from build123d import *

# Parameters (mm, degrees)
SKETCH1_R           = 3
BOSS_EXTRUDE1_DEPTH = 3.7
SKETCH1_3_R         = 1.6
BOSS_EXTRUDE2_DEPTH = 1
SKETCH5_R           = 1.5
BOSS_EXTRUDE3_DEPTH = 1
SKETCH6_R           = 2
BOSS_EXTRUDE4_DEPTH = 1
SKETCH8_R           = 1.5
BOSS_EXTRUDE5_DEPTH = 2.5
SKETCH10_R          = 1.8
BOSS_EXTRUDE6_DEPTH = 1
SKETCH12_R          = 1.65
CUT_EXTRUDE1_DEPTH  = 2


with BuildPart() as part:
    # Sketch1 → Boss-Extrude1 (new body)
    with BuildSketch(Plane(origin=(0, 0, 0), x_dir=(1, 0, 0), z_dir=(0, 1, 0))):
        with Locations((-0.522013312, 0.511138034)):
            Circle(SKETCH1_R)
    extrude(amount=BOSS_EXTRUDE1_DEPTH)

    # Sketch1<3> → Boss-Extrude2 (add)
    with BuildSketch(Plane(origin=(0, 0, 0), x_dir=(1, 0, 0), z_dir=(0, 1, 0))):
        with Locations((-0.522013312, 0.511138034)):
            Circle(SKETCH1_3_R)
    extrude(amount=BOSS_EXTRUDE2_DEPTH)

    # Sketch5 → Boss-Extrude3 (add)
    with BuildSketch(Plane.XZ):
        with Locations((-0.522013312, -0.511138034)):
            Circle(SKETCH5_R)
    extrude(amount=BOSS_EXTRUDE3_DEPTH)

    # Sketch6 → Boss-Extrude4 (add)
    with BuildSketch(Plane.XZ.offset(1)):
        with Locations((-0.522013312, -0.511138034)):
            Circle(SKETCH6_R)
    extrude(amount=BOSS_EXTRUDE4_DEPTH)

    # Sketch8 → Boss-Extrude5 (add)
    with BuildSketch(Plane(origin=(0, -2, 0), x_dir=(-1, 0, 0), z_dir=(0, -1, 0))):
        with Locations((0.522013312, 0.511138034)):
            Circle(SKETCH8_R)
    extrude(amount=BOSS_EXTRUDE5_DEPTH)

    # Sketch10 → Boss-Extrude6 (add)
    with BuildSketch(Plane.XZ.offset(4.5)):
        with Locations((-0.522013312, -0.511138034)):
            Circle(SKETCH10_R)
    extrude(amount=-BOSS_EXTRUDE6_DEPTH)

    # Sketch12 → Cut-Extrude1 (cut)
    with BuildSketch(Plane(origin=(0, 3.7, 0), x_dir=(1, 0, 0), z_dir=(0, 1, 0))):
        with Locations((-0.522013312, 0.511138034)):
            Circle(SKETCH12_R)
    extrude(amount=-CUT_EXTRUDE1_DEPTH, mode=Mode.SUBTRACT)


solid = part.part
Model file for the job. Use its own axes, mm. A direction names the side the tool comes from. Give positions to 0.01 mm unless a question says otherwise; leave off trailing zeros. Loops run counter-clockwise (first coordinate to the right, second up) from the corner with the lowest first, then second, coordinate; pieces in that order, holes last. Notation, with made-up numbers: (24.25, 57.25) -> (50.25, 57.25) arc R17 cw to (50.25, 61.25) -> close; hole circle Ø5 at (0.5, 80.5). An arc over 180 degrees is marked (long way). Use a Markdown table: item, result. Add a question column.
(1) Slice it at D-D on y = -1.75. List the corners of the cut face in (x, z), and give its area (3 significant figures).
(2) Slice it at B-B on z = -1.9. List the corners of the cut face in (x, y).
(3) Drop flat-ended pins along their axis: pin 1 Ø1.6 at (x, z) = (-1, 0) entering from +Y; pin 2 Ø3 at (x, y) = (-3, 1.5) entering from +Z (3 decimals). Give the stop position or say it passes through.
(4) Wall check: line 1 along Y through (x, z) = (-1.9, 1.2); line 2 along X through (y, z) = (2.25, 0.3); line 3 along Y through (x, z) = (0.1, -1.5). Give the ranges that are in metal, low to high.
(5) Tool access for faces 1 (the flat face through (1, 3.7, 1)), 2 (the cylindrical face through (1.325, -1.493, -1.277)), 3 (the cylindrical face through (0.91, -0.49, -0.06)), 4 (the cylindrical face through (1.002, 2.714, 0.121)): list every direction of +Z, -Z, +X, -X, +Y, -Y with a clear straight run to the whole face (end or side of a thin tool).
(6) Slice it at C-C on y = 2.75. List the corners of the cut face in (x, z), and give its area (3 significant figures).
(7) Slice it at A-A on x = -0.25. List the corners of the cut face in (y, z), and give its area (3 significant figures).
(8) Mould opens along Z. For faces 5 (the flat face through (1, 0, 1)), 6 (the flat face through (-1, 1.7, -1)), 7 (the cylindrical face through (-0.197, -2.74, 0.953)) say: +Z half, -Z half, draft (parallel to the pull), parting line (faces both ways), or undercut.
Filled sheet:
| question | item | result |
|---|---|---|
| 1 | outline | circle Ø4 at (-0.52, -0.51) |
| 1 | area | 12.6 mm2 |
| 2 | outline | (-3.18, 0) -> (-1.09, 0) -> (-1.09, -1) -> (-1.96, -1) -> (-1.96, -2) -> (-1.09, -2) -> (-1.09, -3.5) -> (-1.67, -3.5) -> (-1.67, -4.5) -> (0.62, -4.5) -> (0.62, -3.5) -> (0.04, -3.5) -> (0.04, -2) -> (0.92, -2) -> (0.92, -1) -> (0.04, -1) -> (0.04, 0) -> (2.14, 0) -> (2.14, 3.7) -> (0.37, 3.7) -> (0.37, 1.7) -> (-1.41, 1.7) -> (-1.41, 3.7) -> (-3.18, 3.7) -> close |
| 3 | pin 1 | y = 1.7 |
| 3 | pin 2 | z = 2.325 |
| 4 | line 1 | 0 to 3.7 |
| 4 | line 2 | -3.41 to -1.96, 0.91 to 2.37 |
| 4 | line 3 | -4.5 to 1.7 |
| 5 | face 1 | +Z, -Z, +X, -X, +Y |
| 5 | face 2 | -Y |
| 5 | face 3 | none |
| 5 | face 4 | +Y |
| 6 | outline | circle Ø6 at (-0.52, -0.51); hole circle Ø3.3 at (-0.52, -0.51) |
| 6 | area | 19.7 mm2 |
| 7 | outline | (-4.5, -2.29) -> (-3.5, -2.29) -> (-3.5, -1.99) -> (-2, -1.99) -> (-2, -2.49) -> (-1, -2.49) -> (-1, -1.99) -> (0, -1.99) -> (0, -3.5) -> (3.7, -3.5) -> (3.7, -2.14) -> (1.7, -2.14) -> (1.7, 1.12) -> (3.7, 1.12) -> (3.7, 2.48) -> (0, 2.48) -> (0, 0.96) -> (-1, 0.96) -> (-1, 1.47) -> (-2, 1.47) -> (-2, 0.96) -> (-3.5, 0.96) -> (-3.5, 1.27) -> (-4.5, 1.27) -> close |
| 7 | area | 30.5 mm2 |
| 8 | face 5 | draft |
| 8 | face 6 | undercut |
| 8 | face 7 | parting line |
